Source: CAD feature listing. Evaluate the final solid. Frame: model axes, mm. Face numbers are marked on the shaded views. A direction names the side the tool comes from. Coordinates: 2 decimals unless noted, no trailing zeros. Write each loop counter-clockwise with the first axis right and the second up, starting at its lowest first coordinate (ties: lowest second). Pieces come first, ordered by that corner, then holes. Notation, with made-up numbers: (87.25, 86.5) -> (95.25, 86.5) arc R19 ccw to (95.25, 105.5) -> close; hole circle Ø1 at (42, -8). An arc over 180 degrees is marked (long way). One line per item, written item: value. Start each with the question number.
1. First-contact query: P1, Ø10, axis at y = 15, z = -27.5, coming from the -X side; P2, Ø3, axis at x = 26, z = -26, coming from the +Y side; P3, Ø9.5, axis at x = 20.5, y = 8.5, coming from the -Z side. Flat tips, straight axial feed; report the tip coordinate or a pass-through.
2. Line query: line 1 (X direction, y = 9.75, z = -9.5); line 2 (Y direction, x = 29.5, z = -0.6); line 3 (Y direction, x = 29.5, z = -0.35). Output: solid intervals per line, ascending.
3. Access query for the marked faces 5 and 6. Directions: +Z, -Z, +X, -X, +Y, -Y. A direction counts if a zero-diameter tool reaches every point of the face in a straight line with its end or side. Return the directions, or none.
4. Section query A-A, the plane y = 15. Output: boundary loops of the cut face in (x, z), and give its area (3 significant figures).
5. Section query C-C, the plane x = 12. Output: boundary loops of the cut face in (y, z).
6. Section query B-B, the plane x = 29.5. Output: boundary loops of the cut face in (y, z).
7. Section query D-D, the plane z = -16. Output: boundary loops of the cut face in (x, y), and give its area (3 significant figures).
8. Mould query, pull axis X, two halves, no side actions, for the marked faces 1, 2, 3 and 4. Classes: released by +X, released by -X, zero draft, split by the parting line, or undercut.
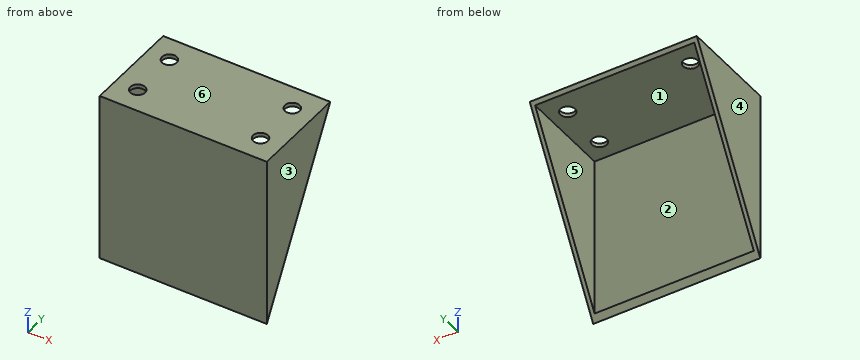
from build123d import *

# Parameters (mm, degrees)
SALIENTE_EXTRUIR3_DEPTH = 34
VACIADO5_T              = -0.8
CROQUIS5_R              = 1.5
CORTAR_EXTRUIR1_DEPTH   = 3


with BuildPart() as part:
    # Croquis4 → Saliente-Extruir3 (new body)
    with BuildSketch(Plane(origin=(0, 0, 0), x_dir=(0, 0, -1), z_dir=(1, 0, 0))):
        Polygon((0, 0), (35, 0), (0, 20), align=None)
    extrude(amount=SALIENTE_EXTRUIR3_DEPTH)

    # Vaciado5
    vaciado5_openings = [part.faces().sort_by_distance(p)[0] for p in [
        (17, 10, -17.5),
    ]]
    offset(amount=VACIADO5_T, openings=vaciado5_openings, kind=Kind.INTERSECTION)

    # Croquis5 → Cortar-Extruir1 (cut)
    with BuildSketch(Plane.XY):
        with Locations((4.5, 15)):
            Circle(CROQUIS5_R)
        with Locations((29.5, 15)):
            Circle(CROQUIS5_R)
        with Locations((29.5, 5)):
            Circle(CROQUIS5_R)
        with Locations((4.5, 5)):
            Circle(CROQUIS5_R)
    extrude(amount=-CORTAR_EXTRUIR1_DEPTH, mode=Mode.SUBTRACT)


solid = part.part
Computed values:
1. P1: passes through
1. P2: stops at y = 0.8
1. P3: stops at z = -0.8
2. line 1: x = 0 to 0.8, 33.2 to 34
2. line 2: y = 0 to 3.5, 6.5 to 13.5, 16.5 to 19.66
2. line 3: y = 0 to 3.5, 6.5 to 13.5, 16.5 to 19.8
3. face 5: -Z, +Y
3. face 6: +Z, +X, -X, +Y, -Y
4. outline: (0, -8.75) -> (0.8, -8.75) -> (0.8, -0.8) -> (3, -0.8) -> (3, 0) -> (0, 0) -> close; (6, -0.8) -> (28, -0.8) -> (28, 0) -> (6, 0) -> close; (31, -0.8) -> (33.2, -0.8) -> (33.2, -8.75) -> (34, -8.75) -> (34, 0) -> (31, 0) -> close
4. area: 35.1 mm²
5. outline: (0, -35) -> (0.8, -33.6) -> (0.8, -0.8) -> (19.54, -0.8) -> (20, 0) -> (0, 0) -> close
6. outline: (0, -35) -> (0.8, -33.6) -> (0.8, -0.8) -> (3.5, -0.8) -> (3.5, 0) -> (0, 0) -> close; (6.5, -0.8) -> (13.5, -0.8) -> (13.5, 0) -> (6.5, 0) -> close; (16.5, -0.8) -> (19.54, -0.8) -> (20, 0) -> (16.5, 0) -> close
7. outline: (0, 0) -> (34, 0) -> (34, 10.86) -> (33.2, 10.86) -> (33.2, 0.8) -> (0.8, 0.8) -> (0.8, 10.86) -> (0, 10.86) -> close
7. area: 43.3 mm²
8. face 1: undercut
8. face 2: undercut
8. face 3: released by +X
8. face 4: released by -X
